Input: dimensioned drawing with shaded views. Units: mm. Origin: part minimum x, y, z. A direction names the side the tool comes from. Coordinates: 2 decimals unless noted, no trailing zeros. Write each loop counter-clockwise with the first axis right and the second up, starting at its lowest first coordinate (ties: lowest second). Pieces come first, ordered by that corner, then holes. Notation, with made-up numbers: (73.25, 28.5) -> (86.25, 28.5) arc R6 cw to (86.25, 36.5) -> close; hole circle Ø8 at (50.5, 43.5). An arc over 180 degrees is marked (long way). One line per item, written item: value. Start each with the question number.
1. First-contact query: P1, Ø5, axis at x = 41, z = 46.5, coming from the -Y side; P2, Ø4, axis at x = 52, z = 44.5, coming from the +Y side; P3, Ø8, axis at x = 11.5, y = 36.5, coming from the -Z side; P4, Ø4, axis at x = 74, y = 2.5, coming from the +Z side. Flat tips, straight axial feed; report the tip coordinate or a pass-through.
2. Section query C-C, the plane y = 46. State how many separate pieces and enclosed holes the cut face has.
3. Line query: line 1 (X direction, y = 3, z = 12.5) (1 decimal); line 2 (Y direction, x = 54.5, z = 6); line 3 (X direction, y = 3.5, z = 49.5). Output: solid intervals per line, ascending.
4. Mould query, pull axis X, two halves, no side actions, for the marked faces 1, 2, 3 and 4. Classes: released by +X, released by -X, zero draft, split by the parting line, or undercut.
5. Section query D-D, the plane z = 60.5. Output: boundary loops of the cut face in (x, y).
6. Access query for the marked faces 5 and 6. Directions: +Z, -Z, +X, -X, +Y, -Y. A direction counts if a zero-diameter tool reaches every point of the face in a straight line with its end or side. Return the directions, or none.
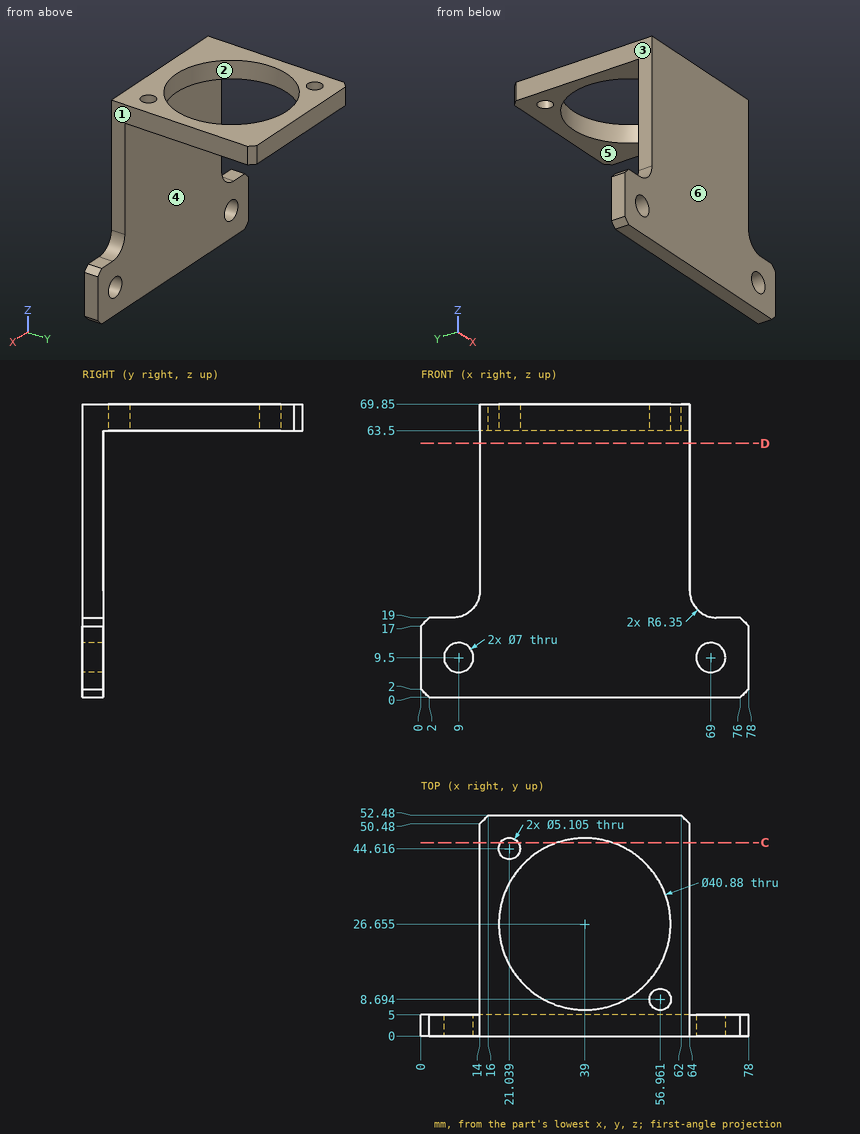
Computed values:
1. P1: stops at y = 0
1. P2: stops at y = 5
1. P3: stops at z = 63.5
1. P4: stops at z = 19
2. separate pieces: 3
2. enclosed holes: 0
3. line 1: x = 0 to 7.2, 10.8 to 67.2, 70.8 to 78
3. line 2: y = 0 to 5
3. line 3: x = 14 to 64
4. face 1: released by +X
4. face 2: undercut
4. face 3: released by -X
4. face 4: zero draft
5. outline: (14, 0) -> (64, 0) -> (64, 5) -> (14, 5) -> close
6. face 5: -Z, +X, -X, +Y
6. face 6: +Z, -Z, +X, -X, -Y
